Read the model definition and answer for the solid it produces. Units are mm, in the model's axes. A direction names the side the tool comes from. Coordinates: 2 decimals unless noted, no trailing zeros. Loops run counter-clockwise (first coordinate to the right, second up) from the corner with the lowest first, then second, coordinate; pieces in that order, holes last.
from build123d import *

# Parameters (mm, degrees)
SKETCH_1_W                   = 60
SKETCH_1_H                   = 60
EXTRUDE_1_DEPTH              = 4
HOLE_WIZARD_M3_1_D           = 3.4
HOLE_WIZARD_M3_1_CSINK_D     = 6.6
HOLE_WIZARD_M3_1_CSINK_ANGLE = 90
HOLE_WIZARD_M3_2_D           = 3.4
HOLE_WIZARD_M3_2_CSINK_D     = 6.6
HOLE_WIZARD_M3_2_CSINK_ANGLE = 90
HOLE_WIZARD_1_D              = 3
SKETCH_9_W                   = 12
SKETCH_9_H                   = 19
SKETCH_9_R                   = 1.5
EXTRUDE_3_DEPTH              = 4
CHAMFER_1_SIZE               = 0.5


with BuildPart() as part:
    # 草图1 → 凸台-拉伸1 (new body)
    with BuildSketch(Plane(origin=(0, 0, 0), x_dir=(1, 0, 0), z_dir=(0, 1, 0))):
        Rectangle(SKETCH_1_W, SKETCH_1_H)
    extrude(amount=EXTRUDE_1_DEPTH)

    # M3 十字槽沉头木螺钉的锥形沉头孔1 (through all)
    with Locations(Plane(origin=(0, 4, 0), x_dir=(1, 0, 0), z_dir=(0, 1, 0))):
        with Locations((-10, 10), (10, 10), (10, -10), (-10, -10)):
            CounterSinkHole(HOLE_WIZARD_M3_1_D / 2, HOLE_WIZARD_M3_1_CSINK_D / 2, counter_sink_angle=HOLE_WIZARD_M3_1_CSINK_ANGLE)

    # M3 十字槽沉头木螺钉的锥形沉头孔2 (through all)
    with Locations(Plane(origin=(0, 0, 0), x_dir=(-1, 0, 0), z_dir=(0, -1, 0))):
        with Locations((19, 0), (0, 0), (-19, 0)):
            CounterSinkHole(HOLE_WIZARD_M3_2_D / 2, HOLE_WIZARD_M3_2_CSINK_D / 2, counter_sink_angle=HOLE_WIZARD_M3_2_CSINK_ANGLE)

    # 孔1 (through all)
    with Locations(Plane(origin=(0, 4, 0), x_dir=(1, 0, 0), z_dir=(0, 1, 0))):
        with Locations((25, 25), (25, -25), (0, -25), (-25, -25), (-25, 25), (0, 25)):
            Hole(HOLE_WIZARD_1_D / 2)

    # 草图9 → 凸台-拉伸3 (add)
    with BuildSketch(Plane(origin=(0, 4, 0), x_dir=(1, 0, 0), z_dir=(0, 1, 0))):
        with Locations((36, -20.5)):
            Rectangle(SKETCH_9_W, SKETCH_9_H)
        with Locations(Location((39, -17, 0), (0, 0, 270))):
            Circle(SKETCH_9_R, mode=Mode.SUBTRACT)
    extrude_3 = extrude(amount=-EXTRUDE_3_DEPTH)

    # 倒角1
    chamfer_1_edges = [part.edges().sort_by_distance(p)[0] for p in [
        (-30, 2, 30),
    ]]
    chamfer(chamfer_1_edges, length=CHAMFER_1_SIZE)

    # 镜向1: 凸台-拉伸3 across plane
    add(extrude_3.mirror(Plane.XY))


solid = part.part
Q1. A cutting plane is placed at D-D (z = -25). Give the vertices of the cut face in (x, y).
Findings below:
outline: (-30, 0) - (-26.5, 0) - (-26.5, 4) - (-30, 4) - close; (-23.5, 0) - (-1.5, 0) - (-1.5, 4) - (-23.5, 4) - close; (1.5, 0) - (23.5, 0) - (23.5, 4) - (1.5, 4) - close; (26.5, 0) - (42, 0) - (42, 4) - (26.5, 4) - close
Q2. Determine the mould class of faces 1 (the face through (6, 2, 30)), 2 (the face through (-17.43, 2.82, 0.65)), 3 (the face through (38.1, 2, -15.8)), 4 (the face through (30, 2, 0)) for opening direction X: +X half, -X half, draft (parallel to the pull), parting line (faces both ways), or undercut.
Findings below:
face 1: draft
face 2: undercut
face 3: undercut
face 4: +X half
Q3. Which of the six approach directions +Z, -Z, +X, -X, +Y, -Y give full straight-line access (tool end or side, diameter ignored) to faces 5 (the face through (-23.89, 1.97, 23.99)), 6 (the face through (36, 2, 11))?
Findings below:
face 5: +Y, -Y
face 6: +X, +Y, -Y
Q4. Flat-ended cylindrical pins translate along their axes: pin 1 Ø2 at (y, z) = (2.5, -1.5) entering from +X; pin 2 Ø2.5 at (x, z) = (39, -17) entering from -Y; pin 3 Ø4.5 at (x, z) = (-19, 0) entering from -Y. Find the tip coordinate at first contact, or state that the pin passes through.
Findings below:
pin 1: stops at x = 30
pin 2: passes through
pin 3: stops at y = 1.05
Q5. A cutting plane is placed at C-C (x = 10). Give the vertices of the cut face in (y, z), then the cut area to 3 significant figures.
Findings below:
outline: (0, -30) - (4, -30) - (4, -13.3) - (2.4, -11.7) - (0, -11.7) - close; (0, -8.3) - (2.4, -8.3) - (4, -6.7) - (4, 6.7) - (2.4, 8.3) - (0, 8.3) - close; (0, 11.7) - (2.4, 11.7) - (4, 13.3) - (4, 30) - (0, 30) - close
area: 208 mm2
Q6. A cutting plane is placed at A-A (x = 0). Give the vertices of the cut face in (y, z).
Findings below:
outline: (0, -30) - (4, -30) - (4, -26.5) - (0, -26.5) - close; (0, -23.5) - (4, -23.5) - (4, -1.7) - (1.6, -1.7) - (0, -3.3) - close; (0, 3.3) - (1.6, 1.7) - (4, 1.7) - (4, 23.5) - (0, 23.5) - close; (0, 26.5) - (4, 26.5) - (4, 30) - (0, 30) - close
Q7. Straight lines are drawn through the part: probe 1 along Z at (x, y) = (25, 2.2); probe 2 along X at (y, z) = (1.95, 25); probe 3 along Z at (x, y) = (-10, 1.3). For each, find the intervals that lie inside material, in ascending order.
Findings below:
probe 1: z = -30 to -26.5, -23.5 to 23.5, 26.5 to 30
probe 2: x = -30 to -26.5, -23.5 to -1.5, 1.5 to 23.5, 26.5 to 42
probe 3: z = -30 to -11.7, -8.3 to 8.3, 11.7 to 30
Q8. A cutting plane is placed at B-B (z = -10). Give the vertices of the cut face in (x, y), then the cut area to 3 significant figures.
Findings below:
outline: (-30, 0) - (-11.7, 0) - (-11.7, 2.4) - (-13.3, 4) - (-30, 4) - close; (-8.3, 0) - (8.3, 0) - (8.3, 2.4) - (6.7, 4) - (-6.7, 4) - (-8.3, 2.4) - close; (11.7, 0) - (30, 0) - (30, 4) - (13.3, 4) - (11.7, 2.4) - close
area: 208 mm2
